from build123d import *

# Parameters (mm, degrees)
SKETCH1_W           = 56
SKETCH1_H           = 45
BOSS_EXTRUDE1_DEPTH = 25
SKETCH2_R           = 5.5
CUT_EXTRUDE1_DEPTH  = 15
SKETCH3_W           = 54
SKETCH3_H           = 43
CUT_EXTRUDE2_DEPTH  = 24
SKETCH4_W           = 15
SKETCH4_H           = 9
CUT_EXTRUDE3_DEPTH  = 24


with BuildPart() as part:
    # Sketch1 → Boss-Extrude1 (new body)
    with BuildSketch(Plane(origin=(0, 0, 0), x_dir=(1, 0, 0), z_dir=(0, 1, 0))):
        Rectangle(SKETCH1_W, SKETCH1_H)
    extrude(amount=BOSS_EXTRUDE1_DEPTH)

    # Sketch2 → Cut-Extrude1 (cut)
    with BuildSketch(Plane.XZ):
        with Locations((-14, 0)):
            Circle(SKETCH2_R)
    extrude(amount=-CUT_EXTRUDE1_DEPTH, mode=Mode.SUBTRACT)

    # Sketch3 → Cut-Extrude2 (cut)
    with BuildSketch(Plane(origin=(0, 25, 0), x_dir=(1, 0, 0), z_dir=(0, 1, 0))):
        Rectangle(SKETCH3_W, SKETCH3_H)
    extrude(amount=-CUT_EXTRUDE2_DEPTH, mode=Mode.SUBTRACT)

    # Sketch4 → Cut-Extrude3 (cut)
    with BuildSketch(Plane(origin=(28, 0, 0), x_dir=(0, 0, -1), z_dir=(1, 0, 0))):
        with Locations((-4, 17.5)):
            Rectangle(SKETCH4_W, SKETCH4_H)
    extrude(amount=-CUT_EXTRUDE3_DEPTH, mode=Mode.SUBTRACT)


solid = part.part
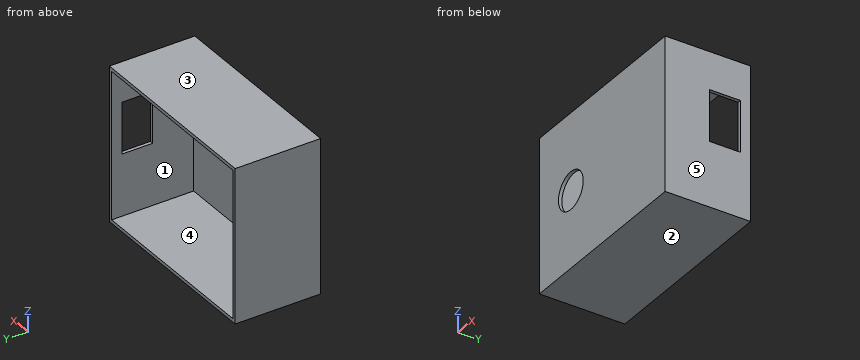
Model file for the job. Use its own axes, mm. Face numbers are marked on the shaded views. A direction names the side the tool comes from. Round coordinates to 2 decimals unless told otherwise and drop trailing zeros. Loops run counter-clockwise (first coordinate to the right, second up) from the corner with the lowest first, then second, coordinate; pieces in that order, holes last. Notation, with made-up numbers: M 41,40.25 L 55,40.25 A27 cw 55,79.25 Z; hole C 34,-22 d10. An arc over 180 degrees is marked long. One line per question, with ' | ' between items.
1) Flat gauge pins, fed straight in: pin 1 (2 mm diameter, centred on x = -7.5, z = -2, fed in from +Y); pin 2 (2 mm diameter, centred on x = 3, z = -4, fed in from -Y). Where does each tip first touch, or does it go through?
Solved:
pin 1: stops at y = 1 | pin 2: stops at y = 0
2) Band-saw the part on A-A (z = 0). Give the cut face in (x, y).
Solved:
outline: M -28,0 L -19.5,0 L -19.5,1 L -27,1 L -27,25 L -28,25 Z; M -8.5,0 L 28,0 L 28,13 L 27,13 L 27,1 L -8.5,1 Z; M 27,22 L 28,22 L 28,25 L 27,25 Z
3) Band-saw the part on B-B (x = -14). Give the cut face in (y, z).
Solved:
outline: M 0,-22.5 L 25,-22.5 L 25,-21.5 L 1,-21.5 L 1,-5.5 L 0,-5.5 Z; M 0,5.5 L 1,5.5 L 1,21.5 L 25,21.5 L 25,22.5 L 0,22.5 Z
4) Mould opens along Z. For the marked faces 3, 4 and 5 say: +Z half, -Z half, draft (parallel to the pull), parting line (faces both ways), or undercut.
Solved:
face 3: +Z half | face 4: undercut | face 5: draft
5) Drill centre lines: line 1 along Z through (x, y) = (18.5, 1.5); line 2 along Z through (x, y) = (-14, 0.65); line 3 along X through (y, z) = (18.75, 18). Where is each one in solid material? Low to high.
Solved:
line 1: z = -22.5 to -21.5, 21.5 to 22.5 | line 2: z = -22.5 to -5.5, 5.5 to 22.5 | line 3: x = -28 to -27, 27 to 28
6) 3-axis set-ups, long thin cutter, end or side, ignore diameter. For the marked faces 1 and 2: which of +Z, -Z, +X, -X, +Y, -Y reach the whole face in a straight line?
Solved:
face 1: +Y | face 2: -Z, +X, -X, +Y, -Y
7) Band-saw the part on C-C (y = 12). Give the cut face in (x, z).
Solved:
outline: M -28,-22.5 L 28,-22.5 L 28,22.5 L -28,22.5 Z; hole M -27,-21.5 L 27,-21.5 L 27,21.5 L -27,21.5 Z
8) Band-saw the part on D-D (z = -18). Give the cut face in (x, y).
Solved:
outline: M -28,0 L 28,0 L 28,25 L 27,25 L 27,1 L -27,1 L -27,25 L -28,25 Z
